from build123d import *

# Parameters (mm, degrees)
SKETCH2_W               = 46
SKETCH2_H               = 42
SKETCH2_W_2             = 26
SKETCH2_H_2             = 22
CUT_EXTRUDE_THIN1_DEPTH = 21.928932188
CHAMFER1_SIZE           = 1


with BuildPart() as part:
    # Sketch1 → Revolve1 (revolve)
    with BuildSketch(Plane(origin=(0, 0, 0), x_dir=(0, 0, -1), z_dir=(1, 0, 0))):
        with BuildLine():
            Line((1009, 0), (1009, 6))
            Line((1009, 6), (1024, 6))
            Line((1024, 6), (1024, 5))
            Line((1024, 5), (1027, 5))
            Line((1027, 5), (1027, 13))
            Line((1027, 13), (1036.171572875, 13))
            ThreePointArc((1036.171572875, 13), (1036.93693974, 12.847759065), (1037.585786438, 12.414213562))
            Line((1037.585786438, 12.414213562), (1046.464466094, 3.535533906))
            ThreePointArc((1046.464466094, 3.535533906), (1047.548329851, 1.913417162), (1047.928932188, 0))
            Line((1047.928932188, 0), (1009, 0))
        make_face()
    revolve(axis=Axis((0, 0, -1178.108206327), (0, 0, 1)))

    # Sketch2 → Cut-Extrude-Thin1 (cut, through all)
    with BuildSketch(Plane.XY.offset(-1027)):
        Rectangle(SKETCH2_W, SKETCH2_H)
        Rectangle(SKETCH2_W_2, SKETCH2_H_2, mode=Mode.SUBTRACT)
    extrude(amount=-CUT_EXTRUDE_THIN1_DEPTH, mode=Mode.SUBTRACT)

    # Chamfer1
    chamfer1_edges = [part.edges().sort_by_distance(p)[0] for p in [
        (0, -6, -1009),
    ]]
    chamfer(chamfer1_edges, length=CHAMFER1_SIZE)


solid = part.part
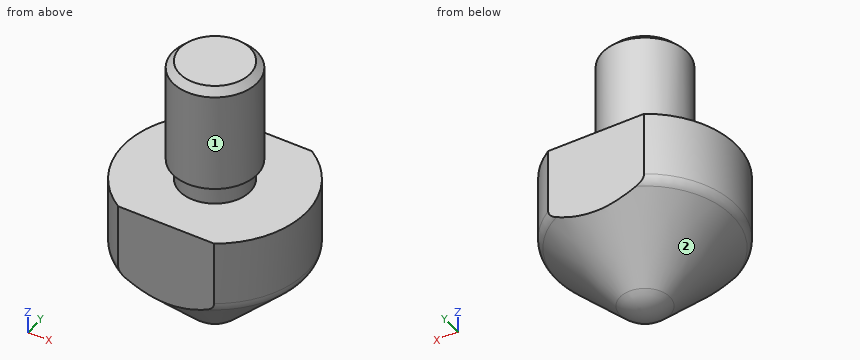
Here's how the part is built. I have some questions about the finished solid (model axes, mm). Face numbers are marked on the shaded views. A direction names the side the tool comes from. Give positions to 0.01 mm unless a question says otherwise; leave off trailing zeros. Loops run counter-clockwise (first coordinate to the right, second up) from the corner with the lowest first, then second, coordinate; pieces in that order, holes last. Notation, with made-up numbers: (61, 0.5) -> (94, 0.5) arc R16 cw to (94, 10.5) -> close; hole circle Ø6 at (78.5, 30). An arc over 180 degrees is marked (long way). One line per item, written item: value.
Q1. If I drill on line 1 along Z through (x, y) = (3.25, 4); line 2 along Y through (x, z) = (-4, -1042); line 3 along Z through (x, y) = (-0.5, -5.25), over which ranges is the centre line in solid material (lowest first)?
Answers follow:
line 1: -1044.85 to -1027, -1024 to -1009.15
line 2: -6.93 to 6.93
line 3: -1044.73 to -1027, -1024 to -1009.27
Q2. Suppose I cut it at D-D on z = -1041.5. Please give me the cut outline in (x, y), then the cut area to 3 significant figures.
Answers follow:
outline: circle Ø17 at (0, 0)
area: 227 mm^2
Q3. I'm going to push flat-ended pins straight in: pin 1 Ø1 at (y, z) = (1, -1019.5) entering from -X; pin 2 Ø12 at (y, z) = (5.5, -1014) entering from +X; pin 3 Ø1.5 at (x, y) = (-7, 6.5) entering from +Z. Where does each tip first touch, or does it pass through?
Answers follow:
pin 1: x = -5.98
pin 2: x = 6
pin 3: z = -1027
Q4. Suppose I cut it at B-B on y = 0. Please give me the cut outline in (x, z), then the cut area to 3 significant figures.
Answers follow:
outline: (-13, -1036.17) arc R2 ccw to (-12.41, -1037.59) -> (-3.54, -1046.46) arc R5 ccw to (3.54, -1046.46) -> (12.41, -1037.59) arc R2 ccw to (13, -1036.17) -> (13, -1027) -> (5, -1027) -> (5, -1024) -> (6, -1024) -> (6, -1010) -> (5, -1009) -> (-5, -1009) -> (-6, -1010) -> (-6, -1024) -> (-5, -1024) -> (-5, -1027) -> (-13, -1027) -> close
area: 632 mm^2
Q5. Suppose I cut it at C-C on z = -1014. Please give me the cut outline in (x, y), then the cut area to 3 significant figures.
Answers follow:
outline: circle Ø12 at (0, 0)
area: 113 mm^2
Q6. Suppose I cut it at A-A on x = 0. Please give me the cut outline in (y, z), then the cut area to 3 significant figures.
Answers follow:
outline: (-11, -1039) -> (-3.54, -1046.46) arc R5 ccw to (3.54, -1046.46) -> (11, -1039) -> (11, -1027) -> (5, -1027) -> (5, -1024) -> (6, -1024) -> (6, -1010) -> (5, -1009) -> (-5, -1009) -> (-6, -1010) -> (-6, -1024) -> (-5, -1024) -> (-5, -1027) -> (-11, -1027) -> close
area: 589 mm^2
Q7. On a 3-axis mill with a long thin cutter (end or side, diameter ignored), from which of +Z, -Z, +X, -X, +Y, -Y can I reach the whole of each face in a straight line? I mean the marked faces 1 and 2. Say none if no direction works.
Answers follow:
face 1: +Z
face 2: -Z
